```python
from build123d import *

# Parameters (mm, degrees)
SKETCH1_W           = 20
SKETCH1_H           = 52
BOSS_EXTRUDE1_DEPTH = 620
SKETCH2_W           = 18
SKETCH2_H           = 50
CUT_EXTRUDE1_DEPTH  = 1200
SKETCH4_R           = 2.75
CUT_EXTRUDE2_DEPTH  = 20
SKETCH5_W           = 1
SKETCH5_H           = 5
CUT_EXTRUDE3_DEPTH  = 1200
SKETCH6_R           = 2.75
CUT_EXTRUDE4_DEPTH  = 20


with BuildPart() as part:
    # Sketch1 → Boss-Extrude1 (new body)
    with BuildSketch(Plane.XY):
        Rectangle(SKETCH1_W, SKETCH1_H)
    extrude(amount=-BOSS_EXTRUDE1_DEPTH)

    # Sketch2 → Cut-Extrude1 (cut)
    with BuildSketch(Plane.XY):
        Rectangle(SKETCH2_W, SKETCH2_H)
    extrude(amount=-CUT_EXTRUDE1_DEPTH, mode=Mode.SUBTRACT)

    # Sketch4 → Cut-Extrude2 (cut)
    with BuildSketch(Plane(origin=(10, 0, 0), x_dir=(0, 0, -1), z_dir=(1, 0, 0))):
        with Locations(Location((15, 0, 0), (0, 0, 90))):
            Circle(SKETCH4_R)
    extrude(amount=-CUT_EXTRUDE2_DEPTH, mode=Mode.SUBTRACT)

    # Sketch5 → Cut-Extrude3 (cut)
    with BuildSketch(Plane.XY):
        with Locations((9.5, 13)):
            Rectangle(SKETCH5_W, SKETCH5_H)
    extrude(amount=-CUT_EXTRUDE3_DEPTH, mode=Mode.SUBTRACT)

    # Sketch6 → Cut-Extrude4 (cut)
    with BuildSketch(Plane(origin=(10, 0, 0), x_dir=(0, 0, -1), z_dir=(1, 0, 0))):
        with Locations(Location((595, 0, 0), (0, 0, 90))):
            Circle(SKETCH6_R)
    extrude(amount=-CUT_EXTRUDE4_DEPTH, mode=Mode.SUBTRACT)


solid = part.part
```
For this review, take the finished solid that the model builds, in its own axes (mm). A direction names the side the tool comes from. Round coordinates to 2 decimals unless told otherwise and drop trailing zeros. Write each loop counter-clockwise with the first axis right and the second up, starting at its lowest first coordinate (ties: lowest second). Pieces come first, ordered by that corner, then holes. Notation, with made-up numbers: (55, -27) - (72, -27) arc R7 ccw to (72, -16) - close; hole circle Ø2 at (46, -7.5). An arc over 180 degrees is marked (long way). Put each result on its own line as item: value.
Q1. Mouldability with a two-part tool opening along Z and no side actions: class faces 1 (the face through (-9.7, 7.8, 0)), 2 (the face through (-9.7, 7.8, -620)), 3 (the face through (0, 26, -306)) as released by +Z, released by -Z, zero draft, split by the parting line, or undercut.
Solved:
face 1: released by +Z
face 2: released by -Z
face 3: zero draft
Q2. We need section A-A (x = -4.75). Give the boundary of the cut face in (y, z).
Solved:
outline: (-26, -620) - (-25, -620) - (-25, 0) - (-26, 0) - close; (25, -620) - (26, -620) - (26, 0) - (25, 0) - close
Q3. Machinability: for faces 4 (the face through (0, -25, -306)), 5 (the face through (-10, 0, -306)), which of the approach directions +Z, -Z, +X, -X, +Y, -Y give a long, thin tool a straight path to every point of the face, cutting with its end or side? Answer none if there is none.
Solved:
face 4: +Z, -Z
face 5: +Z, -Z, -X, +Y, -Y
Q4. Insertion check: pin 1 Ø7 at (y, z) = (0, -595) entering from -X. The pin has a flat end and moves straight along its axis. Give the tip position at first contact, or say it passes through.
Solved:
pin 1: stops at x = -10
Q5. Wall thickness on probe 1 along Z at (x, y) = (-9.3, 0); probe 2 along Y at (x, z) = (9.85, -595); probe 3 along Y at (x, z) = (6, -210): over which ranges is each line inside the solid? List them lowest first.
Solved:
probe 1: z = -620 to -597.75, -592.25 to -17.75, -12.25 to 0
probe 2: y = -26 to -2.75, 2.75 to 10.5, 15.5 to 26
probe 3: y = -26 to -25, 25 to 26
Q6. We need section B-B (z = -491.5). Give the boundary of the cut face in (x, y).
Solved:
outline: (-10, -26) - (10, -26) - (10, 10.5) - (9, 10.5) - (9, -25) - (-9, -25) - (-9, 25) - (9, 25) - (9, 15.5) - (10, 15.5) - (10, 26) - (-10, 26) - close
